Geometry: see drawing. Coordinates: mm, zero at the bounding-box minimum. A direction names the side the tool comes from. Coordinates: 2 decimals unless noted, no trailing zeros. Order: outer loops, then holes, each group sorted by start corner. A loop starts at its lowest first (then second) coordinate and runs counter-clockwise, first axis right, second up.
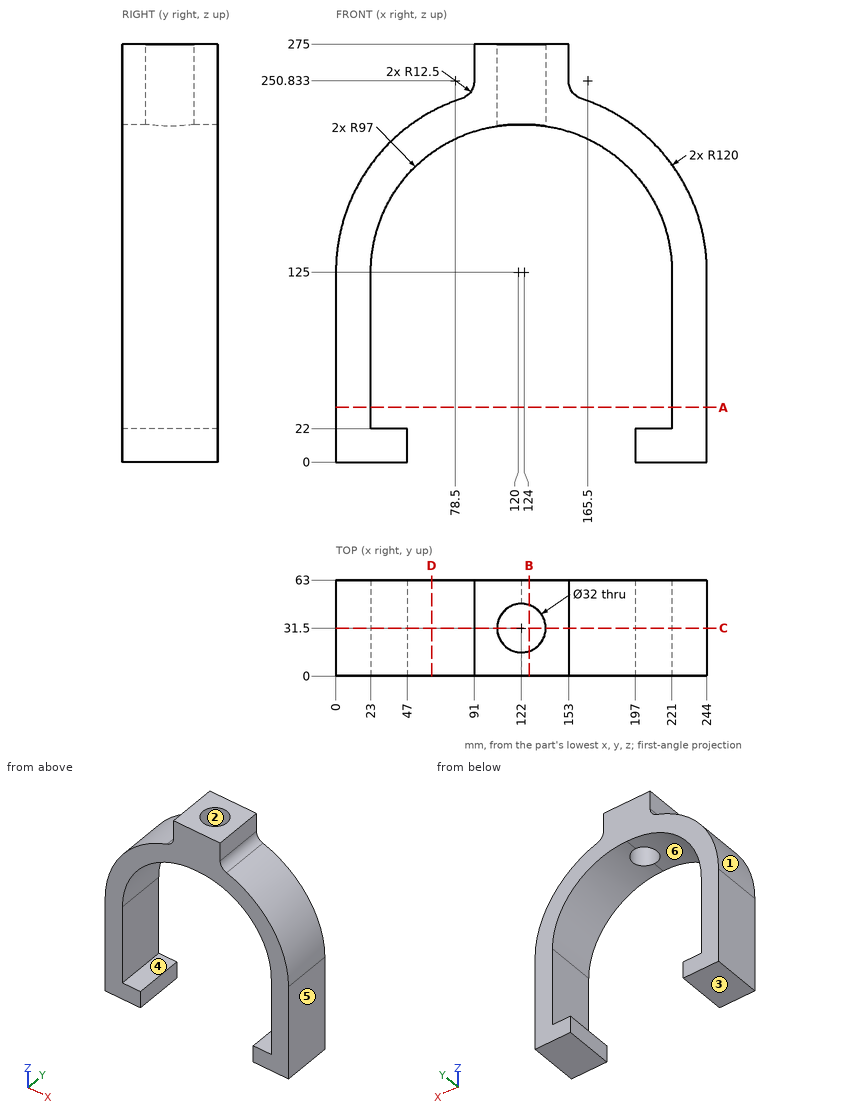
Item 1: Cut plane A-A on z = 36. Return loops of the section in (x, y).
Response values:
outline: (0, 0) - (23, 0) - (23, 63) - (0, 63) - close; (221, 0) - (244, 0) - (244, 63) - (221, 63) - close
Item 2: Draft query along Z for the marked faces 1, 2, 3 and 4. Return one class per face: pulls with the +Z half, pulls with the -Z half, needs draft (parallel to the pull), parting line crosses it, or undercut.
Response values:
face 1: pulls with the +Z half
face 2: needs draft
face 3: pulls with the -Z half
face 4: undercut
Item 3: Cut plane B-B on x = 127. Return loops of the section in (y, z), then the cut area to 3 significant figures.
Response values:
outline: (0, 221.95) - (16.3, 221.95) - (16.3, 275) - (0, 275) - close; (46.7, 221.95) - (63, 221.95) - (63, 275) - (46.7, 275) - close
area: 1,730 mm2
Item 4: Access query for the marked faces 5 and 6. Directions: +Z, -Z, +X, -X, +Y, -Y. A direction counts if a zero-diameter tool reaches every point of the face in a straight line with its end or side. Return the directions, or none.
Response values:
face 5: +Z, -Z, +X, +Y, -Y
face 6: +Y, -Y
Item 5: Pin query (flat end, axial travel): pin 1 Ø6 at (y, z) = (10.5, 181.5) entering from -X; pin 2 Ø3 at (x, y) = (75, 20.5) entering from +Z; pin 3 Ø19.5 at (y, z) = (16.5, 262.5) entering from +X; pin 4 Ø3 at (x, z) = (90.5, 215) entering from -Y. Return the tip coordinate at first contact, or that it passes through.
Response values:
pin 1: stops at x = 12.59
pin 2: stops at z = 236.84
pin 3: stops at x = 153
pin 4: passes through
Item 6: Cut plane C-C on y = 31.5. Return loops of the section in (x, z) (1 decimal).
Response values:
outline: (0, 0) - (47, 0) - (47, 22) - (23, 22) - (23, 125) arc R97 cw to (106, 221) - (106, 275) - (91, 275) - (91, 250.8) arc R12.5 cw to (82.4, 239) arc R120 ccw to (0, 125) - close; (138, 221) arc R97 cw to (221, 125) - (221, 22) - (197, 22) - (197, 0) - (244, 0) - (244, 125) arc R120 ccw to (161.6, 239) arc R12.5 cw to (153, 250.8) - (153, 275) - (138, 275) - close
Item 7: Cut plane D-D on x = 63. Return loops of the section in (y, z).
Response values:
outline: (0, 203.49) - (63, 203.49) - (63, 230.6) - (0, 230.6) - close
Item 8: Ray query, probe 1 along Y at (x, z) = (122, 237); probe 2 along X at (y, z) = (33.5, 88); probe 3 along Z at (x, y) = (44.5, 55). Return the intervals inside material, ascending.
Response values:
probe 1: y = 0 to 15.5, 47.5 to 63
probe 2: x = 0 to 23, 221 to 244
probe 3: z = 0 to 22, 185.9 to 218.27
